Source: three-view drawing plus pictorial views. Frame: mm from the lowest corner of the part. A direction names the side the tool comes from. Give positions to 0.01 mm unless a question says otherwise; leave off trailing zeros. Write each loop counter-clockwise with the first axis right and the second up, starting at its lowest first coordinate (ties: lowest second). Pieces come first, ordered by that corner, then holes. Notation, with made-up numbers: (-21.5, 40.5) -> (10.5, 40.5) arc R14 cw to (10.5, 57.5) -> close; hole circle Ø8 at (26, 19.5). An arc over 180 degrees is marked (long way). Write item = value, one per line.
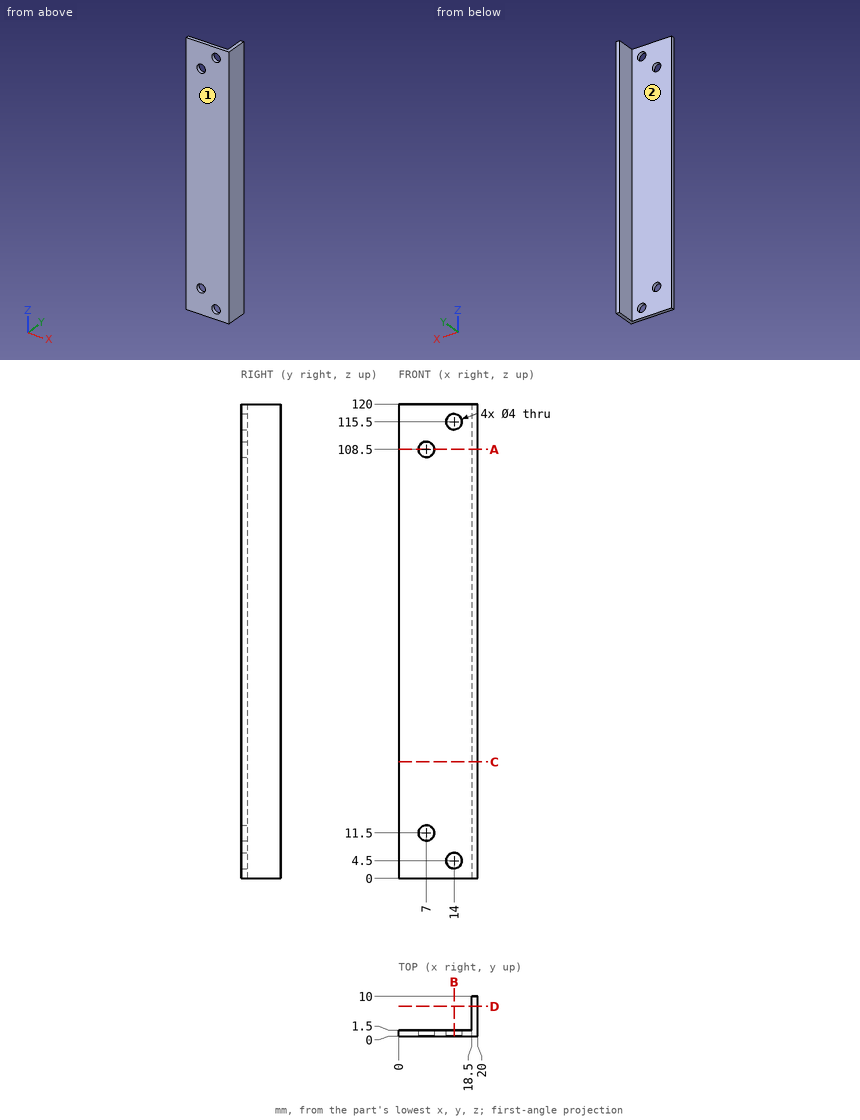
1) Contact query for flat-ended pins moving along their axis: pin 1 (5.5 mm diameter, centred on x = 9.5, z = 78.5, fed in from +Y); pin 2 (3 mm diameter, centred on y = 6.5, z = 60.5, fed in from -X). Output: stop coordinate, or through.
Computed:
pin_1 = 1.5
pin_2 = 18.5
2) Cut plane C-C (z = 29.5). Return the cut outline in (x, y), then the cut area to 4 significant figures.
Computed:
outline = (0, 0) -> (20, 0) -> (20, 10) -> (18.5, 10) -> (18.5, 1.5) -> (0, 1.5) -> close
area = 42.75 mm²
3) Cut plane D-D (y = 7.5). Return the cut outline in (x, z), then the cut area to 3 significant figures.
Computed:
outline = (18.5, 0) -> (20, 0) -> (20, 120) -> (18.5, 120) -> close
area = 180 mm²
4) Material intervals for L1, parallel to Z at x = 7, y = 0.6; L2, parallel to Z at x = 14, y = 0.45; L3, parallel to X at y = 0.7, z = 108.5, sorted ascending.
Computed:
L1 = 0 to 9.5, 13.5 to 106.5, 110.5 to 120
L2 = 0 to 2.5, 6.5 to 113.5, 117.5 to 120
L3 = 0 to 5, 9 to 20
5) Cut plane A-A (z = 108.5). Return the cut outline in (x, y).
Computed:
outline = (0, 0) -> (5, 0) -> (5, 1.5) -> (0, 1.5) -> close; (9, 0) -> (20, 0) -> (20, 10) -> (18.5, 10) -> (18.5, 1.5) -> (9, 1.5) -> close
6) Access query for the marked faces 1 and 2. Directions: +Z, -Z, +X, -X, +Y, -Y. A direction counts if a zero-diameter tool reaches every point of the face in a straight line with its end or side. Return the directions, or none.
Computed:
face_1 = +Z, -Z, +X, -X, -Y
face_2 = +Z, -Z, -X, +Y
7) Cut plane B-B (x = 14). Return the cut outline in (y, z).
Computed:
outline = (0, 0) -> (1.5, 0) -> (1.5, 2.5) -> (0, 2.5) -> close; (0, 6.5) -> (1.5, 6.5) -> (1.5, 113.5) -> (0, 113.5) -> close; (0, 117.5) -> (1.5, 117.5) -> (1.5, 120) -> (0, 120) -> close
